```python
from build123d import *
from build123d.topology import SkipClean

# Parameters (mm, degrees)
SALIENTE_EXTRUIR1_DEPTH                              = 100
SALIENTE_EXTRUIR3_DEPTH                              = 60
CROQUIS8_R                                           = 7
CORTAR_EXTRUIR2_DEPTH                                = 7.5
CORTAR_EXTRUIR3_DEPTH                                = 25
SALIENTE_EXTRUIR5_REACH                              = 169.332
CROQUIS12_W                                          = 116.3
CROQUIS12_H                                          = 2
AVELLANADO_PARA_TORNILLO_CON_CABEZA_2_D              = 3
AVELLANADO_PARA_TORNILLO_CON_CABEZA_2_DEPTH          = 10
AVELLANADO_PARA_TORNILLO_CON_CABEZA_2_CSINK_D        = 5
AVELLANADO_PARA_TORNILLO_CON_CABEZA_2_CSINK_ANGLE    = 90
AVELLANADO_PARA_TORNILLO_CON_CABEZA_2_TIP            = 0.901290929
AVELLANADO_PARA_TORNILLO_CON_CABEZA_2_ON_D           = 3
AVELLANADO_PARA_TORNILLO_CON_CABEZA_2_ON_DEPTH       = 10
AVELLANADO_PARA_TORNILLO_CON_CABEZA_2_ON_CSINK_D     = 5
AVELLANADO_PARA_TORNILLO_CON_CABEZA_2_ON_CSINK_ANGLE = 90
AVELLANADO_PARA_TORNILLO_CON_CABEZA_2_ON_TIP         = 0.901290929
CROQUIS18_R                                          = 10
CROQUIS18_R_2                                        = 3.723403092
CORTAR_EXTRUIR6_DEPTH                                = 10
CROQUIS21_W                                          = 4
CROQUIS21_H                                          = 173.15
SALIENTE_EXTRUIR6_DEPTH                              = 90
CROQUIS22_W                                          = 86
CROQUIS22_H                                          = 172
CORTAR_EXTRUIR7_DEPTH                                = 3
CROQUIS23_W                                          = 3
CROQUIS23_H                                          = 172
CORTAR_EXTRUIR8_DEPTH                                = 2
CORTAR_EXTRUIR9_REACH                                = 195.972
CROQUIS24_W                                          = 3
CROQUIS24_H                                          = 10.09778391
CROQUIS25_W                                          = 116.3
CROQUIS25_H                                          = 2
CORTAR_EXTRUIR10_DEPTH                               = 10


# Read off the part's stored shape, not the designer's step: Recubrir-Lámina1
with BuildPart() as part:
    # Croquis1 → Saliente-Extruir1 (new body)
    with BuildSketch(Plane.XY):
        with BuildLine():
            Line((60, -120), (60, 55))
            ThreePointArc((60, 55), (59.414213562, 56.414213562), (58, 57))
            Line((58, 57), (-58, 57))
            ThreePointArc((-58, 57), (-59.414213562, 56.414213562), (-60, 55))
            Line((-60, 55), (-60, -120))
            Line((-60, -120), (60, -120))
        make_face()
        with BuildLine():
            Line((-57.95, -118), (57.95, -118))
            ThreePointArc((57.95, -118), (58.091421356, -117.941421356), (58.15, -117.8))
            Line((58.15, -117.8), (58.15, 54.95))
            ThreePointArc((58.15, 54.95), (58.091421356, 55.091421356), (57.95, 55.15))
            Line((57.95, 55.15), (-57.95, 55.15))
            ThreePointArc((-57.95, 55.15), (-58.091421356, 55.091421356), (-58.15, 54.95))
            Line((-58.15, 54.95), (-58.15, -117.8))
            ThreePointArc((-58.15, -117.8), (-58.091421356, -117.941421356), (-57.95, -118))
        make_face(mode=Mode.SUBTRACT)
    extrude(amount=SALIENTE_EXTRUIR1_DEPTH)

    # Croquis2 → Saliente-Extruir3 (add, symmetric)
    with BuildSketch(Plane(origin=(0, 0, 0), x_dir=(0, 0, -1), z_dir=(1, 0, 0))):
        Polygon((-51.903464864, 55.258422081), (-20, 0), (-67.842054117, -118.071815959), (-70, -118.071815959), (-22.220404934, -0.154145841), (-54.21286594, 55.258422081), align=None)
    extrude(amount=SALIENTE_EXTRUIR3_DEPTH, both=True)

    # Croquis6 → Revolución1 (revolve)
    with BuildSketch(Plane(origin=(0, 0, 0), x_dir=(0, 0, -1), z_dir=(1, 0, 0)), mode=Mode.PRIVATE) as revoluci_n1_sk:
        Polygon((-24.041451884, 7), (-25.773502692, 10), (-18.294962095, 10), (-18.294962095, 8), (-8.294962095, 8), (-8.294962095, 5), (-23.294962095, 5), (-23.294962095, 7), align=None)
    revolve(revoluci_n1_sk.sketch.rotate(Axis((0, 0, -70), (0, 0, 1)), 90), axis=Axis((0, 0, -70), (0, 0, 1)))

    # Croquis8 → Cortar-Extruir2 (cut, symmetric)
    with SkipClean():  # the faces are left unmerged after this step: merging them gives an invalid solid
        with BuildSketch(Plane.XY.offset(23.294962095)):
            with Locations(Location((0, 0, 0), (0, 0, 154.623066475))):
                Circle(CROQUIS8_R)
        extrude(amount=CORTAR_EXTRUIR2_DEPTH, both=True, mode=Mode.SUBTRACT)

    # Croquis10 → Cortar-Extruir3 (cut, symmetric)
    with BuildSketch(Plane(origin=(0, 0, 0), x_dir=(0, 0, -1), z_dir=(1, 0, 0))):
        Polygon((-29.700523202, 12.801799046), (-22.675993136, 0.634956072), (-22.220404934, -0.154145841), (-27.761841087, -13.830135337), (-29.486165756, -12.415050666), align=None)
    extrude(amount=CORTAR_EXTRUIR3_DEPTH, both=True, mode=Mode.SUBTRACT)

    # Saliente-Extruir5: up to this plane
    saliente_extruir5_end = Plane(origin=(60, 0, 20), z_dir=(0, 0.3755372500045795, 0.9268073013625854))
    # Croquis12 → Saliente-Extruir5 (add, up to the surface)
    with BuildSketch(Plane.XY, mode=Mode.PRIVATE) as saliente_extruir5_sk1:
        with Locations((0, -56.05)):
            Rectangle(CROQUIS12_W, CROQUIS12_H)
    saliente_extruir5_tool1 = split(extrude(saliente_extruir5_sk1.sketch, amount=SALIENTE_EXTRUIR5_REACH, mode=Mode.PRIVATE), bisect_by=saliente_extruir5_end, keep=Keep.BOTH, mode=Mode.PRIVATE)
    add(saliente_extruir5_tool1.solids().sort_by_distance((0, -56.05, 0))[0])

    # Croquis14 → Avellanado para tornillo con cabeza elev (revolve, cut)
    with BuildSketch(Plane(origin=(60, 0, 5), x_dir=(0, 0, -1), z_dir=(0, 1, 0))):
        Polygon((0, 0), (0, 10.901290929), (1.5, 10), (1.5, 1), (2.5, 0), align=None)
    avellanado_para_tornillo_con_cabeza_elev = revolve(axis=Axis((66.35, 0, 5), (-1, 0, 0)), mode=Mode.SUBTRACT)

    # Simetría1: Avellanado para tornillo con cabeza elev across plane
    add(avellanado_para_tornillo_con_cabeza_elev.mirror(Plane(origin=(0, 0, 0), x_dir=(0, 0, 1), z_dir=(1, 0, 0))), mode=Mode.SUBTRACT)

    # Avellanado para tornillo con cabeza  2
    with Locations(Plane(origin=(0, 57, 5), x_dir=(1, 0, 0), z_dir=(0, 1, 0))):
        with Locations((0, 0)):
            CounterSinkHole(AVELLANADO_PARA_TORNILLO_CON_CABEZA_2_D / 2, AVELLANADO_PARA_TORNILLO_CON_CABEZA_2_CSINK_D / 2, depth=AVELLANADO_PARA_TORNILLO_CON_CABEZA_2_DEPTH, counter_sink_angle=AVELLANADO_PARA_TORNILLO_CON_CABEZA_2_CSINK_ANGLE)
            with Locations((0, 0, -(AVELLANADO_PARA_TORNILLO_CON_CABEZA_2_DEPTH + AVELLANADO_PARA_TORNILLO_CON_CABEZA_2_TIP / 2))):  # 118° drill point
                Cone(0, AVELLANADO_PARA_TORNILLO_CON_CABEZA_2_D / 2, AVELLANADO_PARA_TORNILLO_CON_CABEZA_2_TIP, mode=Mode.SUBTRACT)

    # Avellanado para tornillo con cabeza 2 on
    with Locations(Plane(origin=(0, -120, 5), x_dir=(0, 0, -1), z_dir=(0, -1, 0))):
        with Locations((0, 0)):
            CounterSinkHole(AVELLANADO_PARA_TORNILLO_CON_CABEZA_2_ON_D / 2, AVELLANADO_PARA_TORNILLO_CON_CABEZA_2_ON_CSINK_D / 2, depth=AVELLANADO_PARA_TORNILLO_CON_CABEZA_2_ON_DEPTH, counter_sink_angle=AVELLANADO_PARA_TORNILLO_CON_CABEZA_2_ON_CSINK_ANGLE)
            with Locations((0, 0, -(AVELLANADO_PARA_TORNILLO_CON_CABEZA_2_ON_DEPTH + AVELLANADO_PARA_TORNILLO_CON_CABEZA_2_ON_TIP / 2))):  # 118° drill point
                Cone(0, AVELLANADO_PARA_TORNILLO_CON_CABEZA_2_ON_D / 2, AVELLANADO_PARA_TORNILLO_CON_CABEZA_2_ON_TIP, mode=Mode.SUBTRACT)

    # Croquis18 → Cortar-Extruir6 (cut)
    with BuildSketch(Plane(origin=(0, 0, 8.294962095), x_dir=(-1, 0, 0), z_dir=(0, 0, -1))):
        Circle(CROQUIS18_R)
        Circle(CROQUIS18_R_2, mode=Mode.SUBTRACT)
    extrude(amount=-CORTAR_EXTRUIR6_DEPTH, mode=Mode.SUBTRACT)

    # Recubrir-Lámina1 outline → Recubrir-Lámina1 (revolve)
    with BuildSketch(Plane.XZ):
        Polygon((7, 18.294962095), (2.5, 8.294962095), (4.69317122, 8.294962095), (9.19317122, 18.294962095), align=None)
    revolve(axis=Axis((0, 0, 0), (0, 0, 1)))

    # Croquis21 → Saliente-Extruir6 (add)
    with BuildSketch(Plane.XY.offset(100)):
        with Locations((-56.15, -31.425)):
            Rectangle(CROQUIS21_W, CROQUIS21_H)
    extrude(amount=-SALIENTE_EXTRUIR6_DEPTH)

    # Croquis22 → Cortar-Extruir7 (cut)
    with BuildSketch(Plane.ZY.offset(60)):
        with Locations((54.5, -31)):
            Rectangle(CROQUIS22_W, CROQUIS22_H)
    extrude(amount=-CORTAR_EXTRUIR7_DEPTH, mode=Mode.SUBTRACT)

    # Croquis23 → Cortar-Extruir8 (cut)
    with BuildSketch(Plane.ZY.offset(57)):
        with Locations((54.5, -31)):
            Rectangle(CROQUIS23_W, CROQUIS23_H)
    extrude(amount=-CORTAR_EXTRUIR8_DEPTH, mode=Mode.SUBTRACT)

    # Croquis24 → Cortar-Extruir9 (cut, up to next)
    with BuildSketch(Plane.ZY.offset(55), mode=Mode.PRIVATE) as cortar_extruir9_sk1:
        with Locations((54.5, -111.951108045)):
            Rectangle(CROQUIS24_W, CROQUIS24_H)
    cortar_extruir9_tool1 = extrude(cortar_extruir9_sk1.sketch, amount=-CORTAR_EXTRUIR9_REACH, mode=Mode.PRIVATE) & part.part
    add(cortar_extruir9_tool1.solids().sort_by_distance((-55, -111.951108, 54.5))[0], mode=Mode.SUBTRACT)

    # Croquis25 → Cortar-Extruir10 (cut)
    with BuildSketch(Plane(origin=(0, 0, 0), x_dir=(-1, 0, 0), z_dir=(0, 0, -1))):
        with Locations((0, -56.05)):
            Rectangle(CROQUIS25_W, CROQUIS25_H)
    extrude(amount=-CORTAR_EXTRUIR10_DEPTH, mode=Mode.SUBTRACT)


solid = part.part
```
Here's how the part is built. I have some questions about the finished solid (model axes, mm). A direction names the side the tool comes from. Round coordinates to 2 decimals unless told otherwise and drop trailing zeros. Write each loop counter-clockwise with the first axis right and the second up, starting at its lowest first coordinate (ties: lowest second). Pieces come first, ordered by that corner, then holes.
Q1. If we section it at C-C on z = 32: Write out the boundary of the cut face in (x, y).
Q2. If we mould it in two halves opening along Z, with no side actions, what happens to faces 4 (the flat face through (-58, -117, 54)), 5 (the flat face through (1, -57.05, 26)), 6 (the flat face through (-9, -3, 18.295))? For each: +Z half, -Z half, draft (parallel to the pull), parting line (faces both ways), or undercut.
Q3. Which directions (+Z, -Z, +X, -X, +Y, -Y) give clear straight access to the entire face, cutting with the end or side of a thin tool? Please do faces 1 (the flat face through (58.15, -52, 26)), 2 (the flat face through (1, -118, 85)), 3 (the flat face through (-60, -32, 9)).
Q4. If we section it at A-A on z = 75: Write out the boundary of the cut face in (x, y).
Q5. Please list where these lines run through material, in increasing order: probe 1 along Y at (x, z) = (0, 22); probe 2 along X at (y, z) = (-118.2, 5); probe 3 along Y at (x, z) = (-39, 75.5).
Q6. If we section it at D-D on y = -22.5: Write out the boundary of the cut face in (x, z), plus the area to 3 significant figures.
Q7. If we section it at B-B on y = 41.5: Write out the boundary of the cut face in (x, z), plus the area to 3 significant figures.
Q8. Will these pins go through, and if not, where does the flat tip stop? P1, Ø4, axis at y = 6.5, z = 74.5, coming from the -X side; P2, Ø1, axis at x = 19.5, y = -95.5, coming from the +Z side; P3, Ø4, axis at y = 0, z = 5, coming from the -X side.
Answer below:
1. outline: (-60, -120) - (60, -120) - (60, 55) arc R2 ccw to (58, 57) - (-58, 57) arc R2 ccw to (-60, 55) - (-57, 55) - (-57, -117) - (-60, -117) - close; hole (-54.15, -118) - (57.95, -118) arc R0.2 ccw to (58.15, -117.8) - (58.15, -57.05) - (-54.15, -57.05) - close; hole (-54.15, -55.05) - (58.15, -55.05) - (58.15, -29.62) - (-54.15, -29.62) - close; hole (-54.15, -24.29) - (58.15, -24.29) - (58.15, 16.78) - (-54.15, 16.78) - close; hole (-54.15, 20.78) - (58.15, 20.78) - (58.15, 54.95) arc R0.2 ccw to (57.95, 55.15) - (-54.15, 55.15) - close
2. face 4: undercut
2. face 5: draft
2. face 6: -Z half
3. face 1: -Z
3. face 2: +Z
3. face 3: +Z, -Z, -X, +Y, -Y
4. outline: (-60, -120) - (60, -120) - (60, 55) arc R2 ccw to (58, 57) - (-58, 57) arc R2 ccw to (-60, 55) - (-57, 55) - (-57, -117) - (-60, -117) - close; hole (-54.15, -118) - (57.95, -118) arc R0.2 ccw to (58.15, -117.8) - (58.15, 54.95) arc R0.2 ccw to (57.95, 55.15) - (-54.15, 55.15) - close
5. probe 1: y = -120 to -118, -57.05 to -55.05, -10 to -7, 7 to 10, 55.15 to 57
5. probe 2: x = -60 to -1.5, 1.5 to 60
5. probe 3: y = -120 to -118, 55.15 to 57
6. outline: (-60, 0) - (-58.15, 0) - (-58.15, 10) - (-54.15, 10) - (-54.15, 29.12) - (58.15, 29.12) - (58.15, 0) - (60, 0) - (60, 100) - (58.15, 100) - (58.15, 31.27) - (-54.15, 31.27) - (-54.15, 100) - (-60, 100) - (-60, 97.5) - (-57, 97.5) - (-57, 56) - (-55, 56) - (-55, 53) - (-57, 53) - (-57, 11.5) - (-60, 11.5) - close
6. area: 708 mm2
7. outline: (-60, 0) - (-58.15, 0) - (-58.15, 10) - (-54.15, 10) - (-54.15, 43.96) - (58.15, 43.96) - (58.15, 0) - (60, 0) - (60, 100) - (58.15, 100) - (58.15, 46.27) - (-54.15, 46.27) - (-54.15, 100) - (-60, 100) - (-60, 97.5) - (-57, 97.5) - (-57, 56) - (-55, 56) - (-55, 53) - (-57, 53) - (-57, 11.5) - (-60, 11.5) - close
7. area: 725 mm2
8. P1: stops at x = -57
8. P2: stops at z = 61.06
8. P3: stops at x = -59.5
